Source: CAD feature listing. Evaluate the final solid. Frame: model axes, mm. A direction names the side the tool comes from. Give positions to 0.01 mm unless a question says otherwise; leave off trailing zeros. Order: outer loops, then holes, each group sorted by start corner. A loop starts at its lowest first (then second) coordinate and runs counter-clockwise, first axis right, second up.
from build123d import *

# Parameters (mm, degrees)
F0_W     = 50.8
F0_H     = 38.1
F1_DEPTH = 38.1
F2_W     = 19.05
F2_H     = 19.05
F3_DEPTH = 19.05
F4_W     = 19.05
F4_H     = 19.05
F5_DEPTH = 19.05
F7_DEPTH = 31.751
F9_DEPTH = 19.051


with BuildPart() as f1:
    # F0 (on Top) → F1 (new body)
    with BuildSketch(Plane.XY):
        with Locations((25.4, 19.05)):
            Rectangle(F0_W, F0_H)
    extrude(amount=F1_DEPTH)

    # F2 (on face) → F3 (cut)
    with BuildSketch(Plane(origin=(0, 0, 0), x_dir=(0, -1, 0), z_dir=(-1, 0, 0))):
        with Locations((-9.525, 28.575)):
            Rectangle(F2_W, F2_H)
    extrude(amount=-F3_DEPTH, mode=Mode.SUBTRACT)

    # F4 (on face) → F5 (cut)
    with BuildSketch(Plane.YZ.offset(50.8)):
        with Locations((9.525, 28.575)):
            Rectangle(F4_W, F4_H)
    extrude(amount=-F5_DEPTH, mode=Mode.SUBTRACT)

    # F6 (on face) → F7 (cut, through all)
    with BuildSketch(Plane.YZ.offset(31.75)):
        Polygon((0, 38.1), (0, 19.05), (19.05, 38.1), align=None)
    extrude(amount=-F7_DEPTH, mode=Mode.SUBTRACT)

    # F8 (on face) → F9 (cut, through all)
    with BuildSketch(Plane.XZ.offset(-19.05)):
        Polygon((50.8, 38.1), (38.1, 38.1), (50.8, 19.05), align=None)
    extrude(amount=-F9_DEPTH, mode=Mode.SUBTRACT)


solid = f1.part
1) Section query C-C on z = 31. Output: boundary loops of the cut face in (x, y).
Checks:
outline: (0, 19.05) - (19.05, 19.05) - (19.05, 11.95) - (31.75, 11.95) - (31.75, 19.05) - (42.83, 19.05) - (42.83, 38.1) - (0, 38.1) - close
2) Section query A-A on y = 4. Output: boundary loops of the cut face in (x, z).
Checks:
outline: (0, 0) - (50.8, 0) - (50.8, 19.05) - (31.75, 19.05) - (31.75, 23.05) - (19.05, 23.05) - (19.05, 19.05) - (0, 19.05) - close
3) Section query B-B on x = 28.5. Output: boundary loops of the cut face in (y, z).
Checks:
outline: (0, 0) - (38.1, 0) - (38.1, 38.1) - (19.05, 38.1) - (0, 19.05) - close
4) First-contact query: pin 1 Ø3 at (y, z) = (19.5, 26.5) entering from +X; pin 2 Ø9.5 at (y, z) = (9.5, 33.5) entering from -X; pin 3 Ø5.5 at (x, z) = (45, 24) entering from -Y. Flat tips, straight axial feed; report the tip coordinate or a pass-through.
Checks:
pin 1: stops at x = 46.83
pin 2: stops at x = 19.05
pin 3: stops at y = 19.05
5) Section query D-D on y = 31.5. Output: boundary loops of the cut face in (x, z), and give its area (3 significant figures).
Checks:
outline: (0, 0) - (50.8, 0) - (50.8, 19.05) - (38.1, 38.1) - (0, 38.1) - close
area: 1,810 mm2
6) Reachability of faces 1 (the face through (39, 19.05, 26)), 2 (the face through (25, 0, 9)), 3 (the face through (9, 19.05, 28)) from +Z, -Z, +X, -X, +Y, -Y: full face, straight path, thin tool, end or side. Return the list, or none.
Checks:
face 1: +Z, +X, -Y
face 2: +Z, -Z, +X, -X, -Y
face 3: +Z, -X, -Y
7) Ray query, L1, parallel to Z at x = 11, y = 8.5; L2, parallel to X at y = 19, z = 25; L3, parallel to Y at x = 37, z = 34. Return the intervals inside material, ascending.
Checks:
L1: z = 0 to 19.05
L2: x = 19.05 to 31.75
L3: y = 19.05 to 38.1
